Check sheet for the drawn part. Datum: minimum x, y, z corner. Units: mm. A direction names the side the tool comes from. Round coordinates to 2 decimals unless told otherwise and drop trailing zeros. Write each loop counter-clockwise with the first axis right and the second up, starting at its lowest first coordinate (ties: lowest second). Pieces come first, ordered by that corner, then holes. Notation, with made-up numbers: M 68.5,22 L 110.5,22 A28 ccw 110.5,42 Z; hole C 10.25,10.5 d9. An arc over 180 degrees is marked long. One line per item, written item: value. Start each with the question number.
Item 1: Draft check along Y on the marked faces 1, 2 and 3. Enter one of: +Y half, -Y half, draft (parallel to the pull), parting line (faces both ways), or undercut.
Item 2: Thickness scan on probe 1 along Y at (x, z) = (10.5, 5.75); probe 2 along X at (y, z) = (7.25, 5.5); probe 3 along X at (y, z) = (5.5, 3.75). Record the ranges inside material, lowest first. Write a range as from..to.
Item 3: Tool access check on the marked faces 4, 5 and 6. Record the directions out of +Z, -Z, +X, -X, +Y, -Y that give a thin tool (end or side, any length) a straight path to the whole face; none if there is none.
Item 4: Section check A-A, the plane z = 4.25. Record the cut outline in (x, y).
Item 5: Section check B-B, the plane x = 22.5. Record the cut outline in (y, z).
Item 6: Gauge pin test, flat ends, axial feed: pin 1 (1.5 mm diameter, centred on x = 11, y = 4.5, fed in from -Z); pin 2 (0.7 mm diameter, centred on x = 2, z = 3.5, fed in from -Y); pin 3 (1.5 mm diameter, centred on x = 5.5, z = 1.5, fed in from -Y). Record the tip position at first contact, or that the pin passes through.
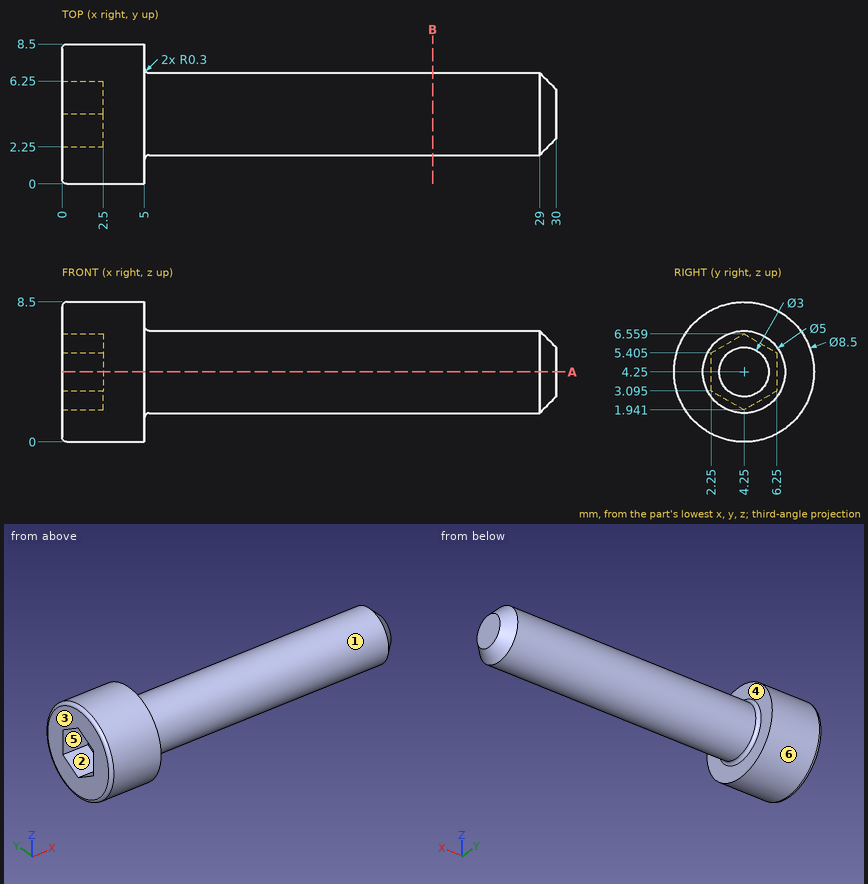
Response values:
1. face 1: parting line
1. face 2: undercut
1. face 3: draft
2. probe 1: y = 2.25..6.25
2. probe 2: x = 0..5
2. probe 3: x = 2.5..30
3. face 4: +X
3. face 5: -X
3. face 6: +X, -X
4. outline: M 0,0.3 A0.3 ccw 0.3,0 L 5,0 L 5,1.45 A0.3 cw 5.3,1.75 L 29,1.75 L 30,2.75 L 30,5.75 L 29,6.75 L 5.3,6.75 A0.3 cw 5,7.05 L 5,8.5 L 0.3,8.5 A0.3 ccw 0,8.2 L 0,6.25 L 2.5,6.25 L 2.5,2.25 L 0,2.25 Z
5. outline: C 4.25,4.25 d5
6. pin 1: stops at z = 1.75
6. pin 2: stops at y = 0.02
6. pin 3: stops at y = 0.61
